Autodesk Fusion 360 part; units mm, degrees
sketch "Sketch1" plane through (0, 0, 0) normal (0, 0, 1) x (1, 0, 0)
  line L0 (38.5, 25) -> (80, 25)
  line L1 (80, 25) -> (80, 11.6)
  line L2 (80, 11.6) -> (38.5, 11.6)
  line L3 (38.5, 11.6) -> (38.5, 25)
  dimension "d1" = 41.5
  dimension "d2" = 13.4
extrude "Extrude1" add sketch "Sketch1" along normal blind 0.6
sketch "Sketch2" plane through (0, 0, 0.6) normal (0, 0, 1) x (-1, 0, 0)
  line L0 (-38.5, -11.6) -> (-80, -11.6)
  line L1 (-80, -11.6) -> (-80, -25)
  line L2 (-80, -25) -> (-38.5, -25)
  line L3 (-38.5, -25) -> (-38.5, -11.6)
  line L4 (-39.5, -24) -> (-79, -24)
  line L5 (-79, -12.6) -> (-39.5, -12.6)
  line L6 (-39.5, -12.6) -> (-39.5, -24)
  line L7 (-80, -18.3) -> (-38.5, -18.3) construction
  line L8 (-66.5, -24) -> (-66.5, -25)
  line L9 (-79, -24) -> (-79, -12.6)
  line L10 (-59.25, -25) -> (-59.25, -11.6) construction
  line L11 (-66.5, -12.6) -> (-66.5, -11.6)
  line L12 (-39.5, -24) -> (-38.5, -24)
  line L13 (-39.5, -12.6) -> (-38.5, -12.6)
  line L14 (-79, -12.6) -> (-79, -11.6)
  line L15 (-79, -24) -> (-79, -25)
  dimension "d5" = 1
  dimension "d6" = 1
  dimension "d12" = 27
extrude "Extrude14" add sketch "Sketch2" along normal blind 3 contours L0 L3 L5 L11 L13 | L0 L1 L2 L9 L14 L15 | L2 L3 L4 L8 L12
extrude "Extrude9" add sketch "Sketch2" along normal blind 2 contours L0 L5 L11 L14 | L3 L6 L12 L13 | L2 L4 L8 L15
sketch "Sketch7" plane through (0, 0, 0.6) normal (0, 0, 1) x (-1, 0, 0)
  line L0 (-39.5, -12.6) -> (-79, -12.6)
  line L1 (-79, -12.6) -> (-79, -24)
  line L2 (-79, -24) -> (-39.5, -24)
  line L3 (-66, -24) -> (-39.5, -24)
  line L4 (-39.5, -24) -> (-39.5, -12.6)
  line L5 (-39.5, -12.6) -> (-66, -12.6)
  line L6 (-66, -12.6) -> (-66, -24)
  line L7 (-39.5, -24) -> (-39.5, -12.6)
extrude "Extrude17" add sketch "Sketch7" along normal blind 1 contours L0 L2 L3 L4 L5 L6 L7
Model file for the job. Use its own axes, mm. A direction names the side the tool comes from. Coordinates: 2 decimals unless noted, no trailing zeros. Write each loop counter-clockwise with the first axis right and the second up, starting at its lowest first coordinate (ties: lowest second). Pieces come first, ordered by that corner, then holes. Notation, with made-up numbers: (15.25, 81) -> (66.25, 81) arc R18 ccw to (66.25, 87) -> close; hole circle Ø9 at (-9.75, 24). An arc over 180 degrees is marked (long way). One line per item, written item: value. Start each with the question number.
1) Slice it at D-D on x = 63.5. Write the cut outline in (y, z), then the cut area to 3 significant figures.
2) Flat gauge pins, fed straight in: pin 1 Ø5.5 at (x, y) = (54.5, 19) entering from +Z; pin 2 Ø0.8 at (x, y) = (74.5, 24.5) entering from +Z; pin 3 Ø2 at (x, y) = (74, 18) entering from +Z. Where does each tip first touch, or does it go through?
3) Slice it at A-A on z = 3.2. Write the cut outline in (x, y), then the cut area to 3 significant figures.
4) Probe probe 1 along X at (y, z) = (15.25, 2.5); probe 2 along X at (y, z) = (14.75, 1.35); probe 3 along Y at (x, z) = (48, 1.7). List the from-to ranges inside material, lowest first.
5) Slice it at B-B on y = 21.5. Write the cut outline in (x, z), then the cut area to 3 significant figures.
6) Slice it at C-C on x = 69.5. Write the cut outline in (y, z), then the cut area to 3 significant figures.
7) Pull direction X, two halves, no side cores. Call faces 1 (the face through (39, 18, 2.6)), 2 (the face through (38.5, 18, 1)), 3 (the face through (66.5, 24.5, 3.1)): +X half, -X half, draft (parallel to the pull), parting line (faces both ways), or undercut.
8) Which spindle directions (+Z, -Z, +X, -X, +Y, -Y) get a long thin tool onto all of the face, cutting with end or side? Do faces 4 (the face through (66.5, 12, 3)), 5 (the face through (39.5, 18, 2)), 6 (the face through (59, 25, 2)). Say none if no direction does.
Answers follow:
1. outline: (11.6, 0) -> (25, 0) -> (25, 3.6) -> (24, 3.6) -> (24, 1.6) -> (12.6, 1.6) -> (12.6, 3.6) -> (11.6, 3.6) -> close
1. area: 25.4 mm2
2. pin 1: z = 1.6
2. pin 2: z = 2.6
2. pin 3: z = 0.6
3. outline: (38.5, 11.6) -> (66.5, 11.6) -> (66.5, 12.6) -> (38.5, 12.6) -> close; (38.5, 24) -> (66.5, 24) -> (66.5, 25) -> (38.5, 25) -> close; (79, 11.6) -> (80, 11.6) -> (80, 25) -> (79, 25) -> close
3. area: 69.4 mm2
4. probe 1: 38.5 to 39.5, 79 to 80
4. probe 2: 38.5 to 66, 79 to 80
4. probe 3: 11.6 to 12.6, 24 to 25
5. outline: (38.5, 0) -> (80, 0) -> (80, 3.6) -> (79, 3.6) -> (79, 0.6) -> (66, 0.6) -> (66, 1.6) -> (39.5, 1.6) -> (39.5, 2.6) -> (38.5, 2.6) -> close
5. area: 56.4 mm2
6. outline: (11.6, 0) -> (25, 0) -> (25, 2.6) -> (24, 2.6) -> (24, 0.6) -> (12.6, 0.6) -> (12.6, 2.6) -> (11.6, 2.6) -> close
6. area: 12.0 mm2
7. face 1: draft
7. face 2: -X half
7. face 3: undercut
8. face 4: +Z, +Y, -Y
8. face 5: +Z
8. face 6: +Z, -Z, +X, -X, +Y
